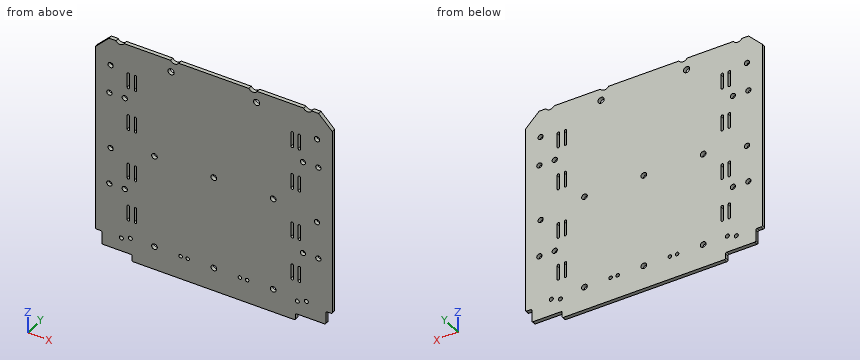
```python
from build123d import *

# Parameters (mm, degrees)
GENERICCARDPCBDEFINITION_START = -0.8
GENERICCARDPCBDEFINITION_DEPTH = 1.6
SKETCH7_R                      = 1.1
SKETCH7_R_2                    = 1.2
SKETCH7_R_3                    = 1.3
SKETCH7_R_4                    = 0.85
SKETCH7_R_5                    = 0.75
CUT_EXTRUDE1_DEPTH             = 1.6


# Read off the part's stored shape, not the designer's step: GenericCardPCBDefinition
with BuildPart() as part:
    # GenericCardPCBDefinition outline → GenericCardPCBDefinition (new body)
    with BuildSketch(Plane(origin=(0, 0, 0), x_dir=(1, 0, 0), z_dir=(0, 1, 0)).offset(GENERICCARDPCBDEFINITION_START)):
        with BuildLine():
            Line((-49.9, -39), (-44.1, -44.8))
            Line((-44.1, -44.8), (-41.232050808, -44.8))
            ThreePointArc((-41.232050808, -44.8), (-39.5, -43.8), (-37.767949192, -44.8))
            Line((-37.767949192, -44.8), (-18.232050808, -44.8))
            ThreePointArc((-18.232050808, -44.8), (-16.5, -43.8), (-14.767949192, -44.8))
            Line((-14.767949192, -44.8), (14.767949192, -44.8))
            ThreePointArc((14.767949192, -44.8), (16.5, -43.8), (18.232050808, -44.8))
            Line((18.232050808, -44.8), (37.767949192, -44.8))
            ThreePointArc((37.767949192, -44.8), (39.5, -43.8), (41.232050808, -44.8))
            Line((41.232050808, -44.8), (44.1, -44.8))
            Line((44.1, -44.8), (49.9, -39))
            Line((49.9, -39), (49.9, 40.7))
            ThreePointArc((49.9, 40.7), (49.753553391, 41.053553391), (49.4, 41.2))
            Line((49.4, 41.2), (47.65, 41.2))
            ThreePointArc((47.65, 41.2), (47.296446609, 41.346446609), (47.15, 41.7))
            Line((47.15, 41.7), (47.15, 46.4))
            ThreePointArc((47.15, 46.4), (47.003553391, 46.753553391), (46.65, 46.9))
            Line((46.65, 46.9), (34.9, 46.9))
            ThreePointArc((34.9, 46.9), (34.546446609, 47.046446609), (34.4, 47.4))
            Line((34.4, 47.4), (34.4, 49.3))
            ThreePointArc((34.4, 49.3), (34.253553391, 49.653553391), (33.9, 49.8))
            Line((33.9, 49.8), (-33.9, 49.8))
            ThreePointArc((-33.9, 49.8), (-34.253553391, 49.653553391), (-34.4, 49.3))
            Line((-34.4, 49.3), (-34.4, 47.4))
            ThreePointArc((-34.4, 47.4), (-34.546446609, 47.046446609), (-34.9, 46.9))
            Line((-34.9, 46.9), (-46.65, 46.9))
            ThreePointArc((-46.65, 46.9), (-47.003553391, 46.753553391), (-47.15, 46.4))
            Line((-47.15, 46.4), (-47.15, 41.7))
            ThreePointArc((-47.15, 41.7), (-47.296446609, 41.346446609), (-47.65, 41.2))
            Line((-47.65, 41.2), (-49.4, 41.2))
            ThreePointArc((-49.4, 41.2), (-49.753553391, 41.053553391), (-49.9, 40.7))
            Line((-49.9, 40.7), (-49.9, -39))
        make_face()
    extrude(amount=GENERICCARDPCBDEFINITION_DEPTH)

    # Sketch7 → Cut-Extrude1 (cut)
    with BuildSketch(Plane(origin=(0, 0.8, 0), x_dir=(1, 0, 0), z_dir=(0, 1, 0))):
        with Locations(Location((-37.5, -20.899999999, 0), (0, 0, 270))):
            Circle(SKETCH7_R)
        with Locations(Location((-44, -20.899999999, 0), (0, 0, 270))):
            Circle(SKETCH7_R)
        with Locations(Location((25, 0, 0), (0, 0, 270))):
            Circle(SKETCH7_R_2)
        with Locations(Location((0, 0, 0), (0, 0, 270))):
            Circle(SKETCH7_R_2)
        with Locations(Location((-25, 0, 0), (0, 0, 270))):
            Circle(SKETCH7_R_2)
        with Locations(Location((0, 39.8, 0), (0, 0, 270))):
            Circle(SKETCH7_R_2)
        with Locations(Location((-25, 39.8, 0), (0, 0, 270))):
            Circle(SKETCH7_R_2)
        with Locations(Location((25, 39.8, 0), (0, 0, 270))):
            Circle(SKETCH7_R_2)
        with Locations(Location((18, -39.8, 0), (0, 0, 270))):
            Circle(SKETCH7_R_3)
        with Locations(Location((-18, -39.8, 0), (0, 0, 270))):
            Circle(SKETCH7_R_3)
        with Locations(Location((-37.5, 19.1, 0), (0, 0, 270))):
            Circle(SKETCH7_R)
        with Locations(Location((-44, 19.1, 0), (0, 0, 270))):
            Circle(SKETCH7_R)
        with Locations(Location((44, 19.1, 0), (0, 0, 270))):
            Circle(SKETCH7_R)
        with Locations(Location((37.5, 19.1, 0), (0, 0, 270))):
            Circle(SKETCH7_R)
        with Locations(Location((43.45, 3.3, 0), (0, 0, 270))):
            Circle(SKETCH7_R)
        with Locations(Location((37.5, -20.899999999, 0), (0, 0, 270))):
            Circle(SKETCH7_R)
        with Locations(Location((44, -20.899999999, 0), (0, 0, 270))):
            Circle(SKETCH7_R)
        with Locations(Location((43.45, -33.2, 0), (0, 0, 270))):
            Circle(SKETCH7_R)
        with Locations(Location((38.95, 39.9, 0), (0, 0, 270))):
            Circle(SKETCH7_R_4)
        with Locations(Location((35.15, 41.2, 0), (0, 0, 270))):
            Circle(SKETCH7_R_4)
        with Locations(Location((-35.15, 39.9, 0), (0, 0, 270))):
            Circle(SKETCH7_R_4)
        with Locations(Location((-38.95, 41.2, 0), (0, 0, 270))):
            Circle(SKETCH7_R_4)
        with Locations(Location((14, 39.85, 0), (0, 0, 270))):
            Circle(SKETCH7_R_5)
        with Locations(Location((11, 39.85, 0), (0, 0, 270))):
            Circle(SKETCH7_R_5)
        with Locations(Location((-11, 39.85, 0), (0, 0, 270))):
            Circle(SKETCH7_R_5)
        with Locations(Location((-14, 39.85, 0), (0, 0, 270))):
            Circle(SKETCH7_R_5)
        with Locations(Location((-43.45, 3.3, 0), (0, 0, 270))):
            Circle(SKETCH7_R)
        with Locations(Location((-43.45, -33.2, 0), (0, 0, 270))):
            Circle(SKETCH7_R)
        with BuildLine():
            Line((32.5, -32.1), (32.5, -26.1))
            ThreePointArc((32.5, -26.1), (33, -25.6), (33.5, -26.1))
            Line((33.5, -26.1), (33.5, -32.1))
            ThreePointArc((33.5, -32.1), (33, -32.6), (32.5, -32.1))
        make_face()
        with BuildLine():
            Line((35.5, -32.1), (35.5, -26.1))
            ThreePointArc((35.5, -26.1), (36, -25.6), (36.5, -26.1))
            Line((36.5, -26.1), (36.5, -32.1))
            ThreePointArc((36.5, -32.1), (36, -32.6), (35.5, -32.1))
        make_face()
        with BuildLine():
            Line((35.5, -13.7), (35.5, -7.7))
            ThreePointArc((35.5, -7.7), (36, -7.2), (36.5, -7.7))
            Line((36.5, -7.7), (36.5, -13.7))
            ThreePointArc((36.5, -13.7), (36, -14.2), (35.5, -13.7))
        make_face()
        with BuildLine():
            Line((32.5, -13.7), (32.5, -7.7))
            ThreePointArc((32.5, -7.7), (33, -7.2), (33.5, -7.7))
            Line((33.5, -7.7), (33.5, -13.7))
            ThreePointArc((33.5, -13.7), (33, -14.2), (32.5, -13.7))
        make_face()
        with BuildLine():
            Line((32.5, 32.1), (32.5, 26.1))
            ThreePointArc((32.5, 26.1), (33, 25.6), (33.5, 26.1))
            Line((33.5, 26.1), (33.5, 32.1))
            ThreePointArc((33.5, 32.1), (33, 32.6), (32.5, 32.1))
        make_face()
        with BuildLine():
            Line((35.5, 32.1), (35.5, 26.1))
            ThreePointArc((35.5, 26.1), (36, 25.6), (36.5, 26.1))
            Line((36.5, 26.1), (36.5, 32.1))
            ThreePointArc((36.5, 32.1), (36, 32.6), (35.5, 32.1))
        make_face()
        with BuildLine():
            Line((35.5, 13.7), (35.5, 7.7))
            ThreePointArc((35.5, 7.7), (36, 7.2), (36.5, 7.7))
            Line((36.5, 7.7), (36.5, 13.7))
            ThreePointArc((36.5, 13.7), (36, 14.2), (35.5, 13.7))
        make_face()
        with BuildLine():
            Line((32.5, 13.7), (32.5, 7.7))
            ThreePointArc((32.5, 7.7), (33, 7.2), (33.5, 7.7))
            Line((33.5, 7.7), (33.5, 13.7))
            ThreePointArc((33.5, 13.7), (33, 14.2), (32.5, 13.7))
        make_face()
        with BuildLine():
            Line((-32.5, 13.7), (-32.5, 7.7))
            ThreePointArc((-32.5, 7.7), (-33, 7.2), (-33.5, 7.7))
            Line((-33.5, 7.7), (-33.5, 13.7))
            ThreePointArc((-33.5, 13.7), (-33, 14.2), (-32.5, 13.7))
        make_face()
        with BuildLine():
            Line((-35.5, 13.7), (-35.5, 7.7))
            ThreePointArc((-35.5, 7.7), (-36, 7.2), (-36.5, 7.7))
            Line((-36.5, 7.7), (-36.5, 13.7))
            ThreePointArc((-36.5, 13.7), (-36, 14.2), (-35.5, 13.7))
        make_face()
        with BuildLine():
            Line((-35.5, 32.1), (-35.5, 26.1))
            ThreePointArc((-35.5, 26.1), (-36, 25.6), (-36.5, 26.1))
            Line((-36.5, 26.1), (-36.5, 32.1))
            ThreePointArc((-36.5, 32.1), (-36, 32.6), (-35.5, 32.1))
        make_face()
        with BuildLine():
            Line((-32.5, 32.1), (-32.5, 26.1))
            ThreePointArc((-32.5, 26.1), (-33, 25.6), (-33.5, 26.1))
            Line((-33.5, 26.1), (-33.5, 32.1))
            ThreePointArc((-33.5, 32.1), (-33, 32.6), (-32.5, 32.1))
        make_face()
        with BuildLine():
            Line((-32.5, -13.7), (-32.5, -7.7))
            ThreePointArc((-32.5, -7.7), (-33, -7.2), (-33.5, -7.7))
            Line((-33.5, -7.7), (-33.5, -13.7))
            ThreePointArc((-33.5, -13.7), (-33, -14.2), (-32.5, -13.7))
        make_face()
        with BuildLine():
            Line((-35.5, -13.7), (-35.5, -7.7))
            ThreePointArc((-35.5, -7.7), (-36, -7.2), (-36.5, -7.7))
            Line((-36.5, -7.7), (-36.5, -13.7))
            ThreePointArc((-36.5, -13.7), (-36, -14.2), (-35.5, -13.7))
        make_face()
        with BuildLine():
            Line((-35.5, -32.1), (-35.5, -26.1))
            ThreePointArc((-35.5, -26.1), (-36, -25.6), (-36.5, -26.1))
            Line((-36.5, -26.1), (-36.5, -32.1))
            ThreePointArc((-36.5, -32.1), (-36, -32.6), (-35.5, -32.1))
        make_face()
        with BuildLine():
            Line((-32.5, -32.1), (-32.5, -26.1))
            ThreePointArc((-32.5, -26.1), (-33, -25.6), (-33.5, -26.1))
            Line((-33.5, -26.1), (-33.5, -32.1))
            ThreePointArc((-33.5, -32.1), (-33, -32.6), (-32.5, -32.1))
        make_face()
    extrude(amount=-CUT_EXTRUDE1_DEPTH, mode=Mode.SUBTRACT)


solid = part.part
```
Read the model definition and answer for the solid it produces. Units are mm, in the model's axes. Give positions to 0.01 mm unless a question says otherwise; leave off trailing zeros. Order: outer loops, then holes, each group sorted by start corner. A loop starts at its lowest first (then second) coordinate and runs counter-clockwise, first axis right, second up. Notation, with made-up numbers: (-20.75, 77.5) -> (15.25, 77.5) arc R19 ccw to (15.25, 86.5) -> close; hole circle Ø9 at (64.25, 26.25). An arc over 180 degrees is marked (long way). One line per item, written item: value. Start each with the question number.
(1) The part is cut by section B-B (z = 12.5). Determine the outline of the cut face in (x, y), and give its area (3 significant figures).
(2) Flat-ended cylindrical pins translate along their axes: P1, Ø0.5, axis at x = -42.5, y = 0.5, coming from the -Z side; P2, Ø3.5, axis at x = -44, z = 20.9, coming from the -Y side; P3, Ø0.8, axis at y = 0, z = -44, coming from the +X side. Find the tip coordinate at first contact, or state that the pin passes through.
(3) The part is cut by section A-A (z = 0). Determine the outline of the cut face in (x, y).
(4) The part is cut by section C-C (y = -0.5). State how many separate pieces and enclosed holes the cut face has, and give its area (3 significant figures).
(5) Straight lines are drawn through the part: L1, parallel to X at y = 0.3, z = 12.5; L2, parallel to X at y = 0.3, z = 20.9; L3, parallel to Z at x = 42.5, y = 0.2. For each, find the intervals that lie inside material, in ascending order.
Taken from the geometry:
1. outline: (-49.9, -0.8) -> (-36.5, -0.8) -> (-36.5, 0.8) -> (-49.9, 0.8) -> close; (-35.5, -0.8) -> (-33.5, -0.8) -> (-33.5, 0.8) -> (-35.5, 0.8) -> close; (-32.5, -0.8) -> (32.5, -0.8) -> (32.5, 0.8) -> (-32.5, 0.8) -> close; (33.5, -0.8) -> (35.5, -0.8) -> (35.5, 0.8) -> (33.5, 0.8) -> close; (36.5, -0.8) -> (49.9, -0.8) -> (49.9, 0.8) -> (36.5, 0.8) -> close
1. area: 153 mm^2
2. P1: z = -46.9
2. P2: y = -0.8
2. P3: x = 47.15
3. outline: (-49.9, -0.8) -> (-26.2, -0.8) -> (-26.2, 0.8) -> (-49.9, 0.8) -> close; (-23.8, -0.8) -> (-1.2, -0.8) -> (-1.2, 0.8) -> (-23.8, 0.8) -> close; (1.2, -0.8) -> (23.8, -0.8) -> (23.8, 0.8) -> (1.2, 0.8) -> close; (26.2, -0.8) -> (49.9, -0.8) -> (49.9, 0.8) -> (26.2, 0.8) -> close
4. separate pieces: 1
4. enclosed holes: 44
4. area: 9,070 mm^2
5. L1: -49.9 to -36.5, -35.5 to -33.5, -32.5 to 32.5, 33.5 to 35.5, 36.5 to 49.9
5. L2: -49.9 to -45.1, -42.9 to -38.6, -36.4 to 36.4, 38.6 to 42.9, 45.1 to 49.9
5. L3: -46.9 to -3.85, -2.75 to 32.65, 33.75 to 44.8
